Can you work these out from the model? Positions are in its coordinate system, mm. A direction names the side the tool comes from. Give positions to 0.01 mm unless a question says otherwise; leave off trailing zeros. Loops run counter-clockwise (first coordinate to the right, second up) from the corner with the lowest first, then second, coordinate; pieces in that order, holes last. Notation, with made-up numbers: (57, 24) -> (97, 24) arc R22 ccw to (97, 31) -> close; hole circle Ø3 at (53.5, -15). An arc over 180 degrees is marked (long way). Return JSON: item names as keys, results as strings. Group by question number.
Q1. I need wall thicknesses on line 1 along X through (y, z) = (-4, 3); line 2 along X through (y, z) = (-17, 3.25); line 3 along Y through (x, z) = (-4, 6.5). Which ranges of each line are inside material? Lowest first, please. Write a range as [from, to].
Q2. Suppose I cut it at A-A, the plane z = 6.25. Please give me the cut outline in (x, y), and give its area (3 significant figures).
Q3. Which directions (+Z, -Z, +X, -X, +Y, -Y) give clear straight access to the entire face, cutting with the end or side of a thin tool? Please do faces 1 (the flat face through (-3, -14, 7)), 2 (the flat face through (-6, -18, 3)).
Q4. Will these pins go through, and if not, where does the flat tip stop? pin 1 (4 mm diameter, centred on y = -19.5, z = 3.5, fed in from -X); pin 2 (3.5 mm diameter, centred on y = -17.5, z = 4.5, fed in from -X).
Q5. Suppose I cut it at B-B, the plane y = -7. Please give me the cut outline in (x, z), and give its area (3 significant figures).
```python
from build123d import *

# Parameters (mm, degrees)
BOSS_EXTRU_2_DEPTH = 7
CONG_1_R           = 7
CONG_2_R           = 15


with BuildPart() as part:
    # Esquisse1 → Boss.-Extru.2 (new body)
    with BuildSketch(Plane.XY):
        with BuildLine():
            Line((-5, 0), (-5, -10.5))
            Line((-5, -10.5), (-6, -14.5))
            Line((-6, -14.5), (-6, -21.5))
            ThreePointArc((-6, -21.5), (-4.822875656, -27.189860092), (0, -23.949489743))
            Line((0, -23.949489743), (0, 0))
            Line((0, 0), (-5, 0))
        make_face()
    extrude(amount=BOSS_EXTRU_2_DEPTH)

    # Congé1
    cong_1_edges = [part.edges().sort_by_distance(p)[0] for p in [
        (-6, -21.5, 3.5),
    ]]
    fillet(cong_1_edges, radius=CONG_1_R)

    # Congé2
    cong_2_edges = [part.edges().sort_by_distance(p)[0] for p in [
        (-6, -14.5, 3.5),
        (-5, -10.5, 3.5),
    ]]
    fillet(cong_2_edges, radius=CONG_2_R)


solid = part.part
```
Ans:
{
 "1": {"line 1": "x = [-5, 0]", "line 2": "x = [-6, 0]", "line 3": "y = [-27.41, 0]"},
 "2": {"outline": "(-6.67, -22.46) arc R3.5 ccw (long way) to (0, -23.95) -> (0, 0) -> (-5, 0) -> (-5, -8.65) arc R15 cw to (-5.45, -12.29) -> (-5.55, -12.71) arc R15 ccw to (-6, -16.35) -> (-6, -19.48) arc R7 cw to start", "area": "152 mm^2"},
 "3": {"face 1": "+Z, +X, -X, +Y, -Y", "face 2": "+Z, -Z, -X, +Y"},
 "4": {"pin 1": "stops at x = -6.3", "pin 2": "stops at x = -6"},
 "5": {"outline": "(-5, 0) -> (0, 0) -> (0, 7) -> (-5, 7) -> close", "area": "35.0 mm^2"}
}
